```python
from build123d import *

# Parameters (mm, degrees)
SKETCH1_W                = 40
SKETCH1_H                = 40
BOSS_EXTRUDE1_DEPTH      = 40
SKETCH2_W                = 25
SKETCH2_H                = 20
CUT_EXTRUDE1_DEPTH       = 40
CHAMFER1_SIZE            = 15
CUT_EXTRUDE2_DEPTH       = 15
CHAMFER2_SIZE            = 4
SKETCH4_R                = 2.6
CUT_EXTRUDE3_DEPTH       = 17
BOSS_EXTRUDE2_DEPTH      = 8
BOSS_EXTRUDE2_DEPTH_BACK = 40
SKETCH5_W                = 40
SKETCH5_H                = 8.5
SKETCH10_W               = 14
SKETCH10_H               = 10
CUT_EXTRUDE5_DEPTH       = 26
SKETCH8_R                = 5.6
CUT_EXTRUDE4_DEPTH       = 34
BOSS_EXTRUDE3_DEPTH      = 20
FILLET3_R                = 4
FILLET4_R                = 2
CHAMFER7_SIZE            = 25
CHAMFER8_SIZE            = 2
CHAMFER8_SIZE2           = 10
FILLET7_R                = 2
SKETCH14_W               = 40
SKETCH14_H               = 8.5
BOSS_EXTRUDE4_DEPTH      = 15
SKETCH16_W               = 40
SKETCH16_H               = 8.5
BOSS_EXTRUDE5_DEPTH      = 15
SKETCH12_R               = 11.1
CUT_EXTRUDE6_DEPTH       = 4.5
CUT_EXTRUDE7_START       = -7.5
SKETCH13_R               = 11.1
CUT_EXTRUDE7_DEPTH       = 7.5
SKETCH15_R               = 2.1
CUT_EXTRUDE8_DEPTH       = 10
CHAMFER10_SIZE           = 0.5
FILLET8_R                = 8


with BuildPart() as part:
    # Sketch1 → Boss-Extrude1 (new body)
    with BuildSketch(Plane(origin=(0, 0, 0), x_dir=(1, 0, 0), z_dir=(0, 1, 0))):
        with Locations((20, 20)):
            Rectangle(SKETCH1_W, SKETCH1_H)
    extrude(amount=BOSS_EXTRUDE1_DEPTH)

    # Sketch2 → Cut-Extrude1 (cut)
    with BuildSketch(Plane(origin=(0, 40, 0), x_dir=(1, 0, 0), z_dir=(0, 1, 0))):
        with Locations((12.5, 30)):
            Rectangle(SKETCH2_W, SKETCH2_H)
    extrude(amount=-CUT_EXTRUDE1_DEPTH, mode=Mode.SUBTRACT)

    # Chamfer1
    chamfer1_edges = [part.edges().sort_by_distance(p)[0] for p in [
        (0, 20, 0),
    ]]
    chamfer(chamfer1_edges, length=CHAMFER1_SIZE)

    # Sketch3 → Cut-Extrude2 (cut)
    with BuildSketch(Plane.XY):
        Polygon((0, 10), (0, 15), (15, 15), (15, 5), (0, 5), align=None)
        Polygon((0, 30), (0, 25), (15, 25), (15, 35), (0, 35), align=None)
    extrude(amount=-CUT_EXTRUDE2_DEPTH, mode=Mode.SUBTRACT)

    # Chamfer2
    chamfer2_edges = [part.edges().sort_by_distance(p)[0] for p in [
        (15, 35, -7.5),
        (15, 25, -7.5),
        (15, 15, -7.5),
        (15, 5, -7.5),
    ]]
    chamfer(chamfer2_edges, length=CHAMFER2_SIZE)

    # Sketch4 → Cut-Extrude3 (cut)
    with BuildSketch(Plane.XY.offset(-15)):
        with Locations((8, 30)):
            Circle(SKETCH4_R)
        with Locations((8, 10)):
            Circle(SKETCH4_R)
    extrude(amount=-CUT_EXTRUDE3_DEPTH, mode=Mode.SUBTRACT)

    # Sketch5 → Boss-Extrude2 (add, two sides: drawn at the far end of the back side and taken through both)
    with BuildSketch(Plane(origin=(0, 0, -40), x_dir=(-1, 0, 0), z_dir=(0, 0, -1)).offset(-BOSS_EXTRUDE2_DEPTH_BACK)):
        with Locations((-60, 4.25)):
            Rectangle(SKETCH5_W, SKETCH5_H)
        with Locations((-60, 30.25)):
            Rectangle(SKETCH5_W, SKETCH5_H)
    extrude(amount=BOSS_EXTRUDE2_DEPTH + BOSS_EXTRUDE2_DEPTH_BACK)

    # Sketch10 → Cut-Extrude5 (cut)
    with BuildSketch(Plane(origin=(40, 0, 0), x_dir=(0, 0, -1), z_dir=(1, 0, 0))):
        with Locations((29, 20)):
            Rectangle(SKETCH10_W, SKETCH10_H)
    extrude(amount=-CUT_EXTRUDE5_DEPTH, mode=Mode.SUBTRACT)

    # Sketch8 → Cut-Extrude4 (cut)
    with BuildSketch(Plane(origin=(0, 32, 0), x_dir=(1, 0, 0), z_dir=(0, 1, 0))):
        with Locations(Location((65, 38, 0), (0, 0, 270))):
            Circle(SKETCH8_R)
    extrude(amount=-CUT_EXTRUDE4_DEPTH, mode=Mode.SUBTRACT)

    # Sketch9 → Boss-Extrude3 (add)
    with BuildSketch(Plane(origin=(40, 0, 0), x_dir=(0, 0, -1), z_dir=(1, 0, 0))):
        Polygon((0, 40), (0, 55), (4, 55), (20, 40), align=None)
        Polygon((0, 0), (0, -15), (4, -15), (20, 0), align=None)
    extrude(amount=-BOSS_EXTRUDE3_DEPTH)

    # Fillet3
    fillet3_edges = [part.edges().sort_by_distance(p)[0] for p in [
        (20, 55, -2),
        (40, 55, -2),
        (20, -15, -2),
        (40, -15, -2),
    ]]
    fillet(fillet3_edges, radius=FILLET3_R)

    # Fillet4
    fillet4_edges = [part.edges().sort_by_distance(p)[0] for p in [
        (32.5, 40, -40),
        (32.5, 0, -40),
    ]]
    fillet(fillet4_edges, radius=FILLET4_R)

    # Chamfer7
    chamfer7_edges = [part.edges().sort_by_distance(p)[0] for p in [
        (80, 4.25, 0),
        (80, 30.25, 0),
    ]]
    chamfer(chamfer7_edges, length=CHAMFER7_SIZE)

    # Chamfer8
    chamfer8_edges = [part.edges().sort_by_distance(p)[0] for p in [
        (40, 20, -36),
    ]]
    chamfer8_side = [part.faces().sort_by_distance(p)[0] for p in [
        (40, 16.5625, -17.75),
    ]]
    chamfer(chamfer8_edges, length=CHAMFER8_SIZE, length2=CHAMFER8_SIZE2, reference=chamfer8_side[0])

    # Fillet7
    fillet7_edges = [part.edges().sort_by_distance(p)[0] for p in [
        (27.5, 15, -36),
        (32.5, 15, -22),
        (32.5, 25, -22),
        (27.5, 25, -36),
        (35, 25, -37),
        (35, 15, -37),
    ]]
    fillet(fillet7_edges, radius=FILLET7_R)

    # Sketch14 → Boss-Extrude4 (add)
    with BuildSketch(Plane(origin=(0, 0, -48), x_dir=(-1, 0, 0), z_dir=(0, 0, -1))):
        with Locations((-60, 4.25)):
            Rectangle(SKETCH14_W, SKETCH14_H)
    extrude(amount=BOSS_EXTRUDE4_DEPTH)

    # Sketch16 → Boss-Extrude5 (add)
    with BuildSketch(Plane(origin=(0, 0, -48), x_dir=(-1, 0, 0), z_dir=(0, 0, -1))):
        with Locations((-60, 30.25)):
            Rectangle(SKETCH16_W, SKETCH16_H)
    extrude(amount=BOSS_EXTRUDE5_DEPTH)

    # Sketch12 → Cut-Extrude6 (cut)
    with BuildSketch(Plane(origin=(0, 34.5, 0), x_dir=(1, 0, 0), z_dir=(0, 1, 0))):
        with Locations(Location((65, 38, 0), (0, 0, 180))):
            Circle(SKETCH12_R)
    extrude(amount=-CUT_EXTRUDE6_DEPTH, mode=Mode.SUBTRACT)

    # Sketch13 → Cut-Extrude7 (cut)
    with BuildSketch(Plane.XZ.offset(CUT_EXTRUDE7_START)):
        with Locations(Location((65, -38, 0), (0, 0, 180))):
            Circle(SKETCH13_R)
    extrude(amount=CUT_EXTRUDE7_DEPTH, mode=Mode.SUBTRACT)

    # Sketch15 → Cut-Extrude8 (cut)
    with BuildSketch(Plane.XZ):
        with Locations(Location((65.260929409, -54.130501699, 0), (0, 0, 270))):
            Circle(SKETCH15_R)
        with Locations(Location((65.16900186, -21.868239994, 0), (0, 0, 270))):
            Circle(SKETCH15_R)
    extrude(amount=-CUT_EXTRUDE8_DEPTH, mode=Mode.SUBTRACT)

    # Chamfer10
    chamfer10_edges = [part.edges().sort_by_distance(p)[0] for p in [
        (76.1, 34.5, -38),
        (76.1, 0, -38),
    ]]
    chamfer(chamfer10_edges, length=CHAMFER10_SIZE)

    # Fillet8
    fillet8_edges = [part.edges().sort_by_distance(p)[0] for p in [
        (55, 30.25, 0),
        (55, 4.25, 0),
        (80, 4.25, -25),
        (80, 30.25, -25),
        (80, 4.25, -63),
        (40, 4.25, -63),
        (80, 30.25, -63),
        (40, 30.25, -63),
    ]]
    fillet(fillet8_edges, radius=FILLET8_R)


solid = part.part
```
Geometry: final body of the model. Coordinates: model frame, mm. A direction names the side the tool comes from. Round coordinates to 2 decimals unless told otherwise and drop trailing zeros. Loops run counter-clockwise (first coordinate to the right, second up) from the corner with the lowest first, then second, coordinate; pieces in that order, holes last. Notation, with made-up numbers: (67, 89) -> (80, 89) arc R14 ccw to (80, 106) -> close; hole circle Ø5 at (34.25, 51). An arc over 180 degrees is marked (long way). Write each question's results on one line, items separated by ' | '.
Item 1: Pin query (flat end, axial travel): pin 1 Ø2.5 at (x, z) = (65.26, -54.13) entering from -Y; pin 2 Ø5.5 at (x, z) = (5.5, -7.5) entering from +Y; pin 3 Ø6 at (x, y) = (70, -4.5) entering from -Z; pin 4 Ø20 at (x, z) = (64.5, -45.5) entering from -Y. Return the tip coordinate at first contact, or that it passes through.
Answers below:
pin 1: stops at y = 26 | pin 2: stops at y = 40 | pin 3: passes through | pin 4: stops at y = 0
Item 2: Cut plane C-C on x = 69.5. State how many separate pieces and enclosed holes the cut face has, and give its area (3 significant figures).
Answers below:
separate pieces: 4 | enclosed holes: 0 | area: 547 mm²
Item 3: Cut plane D-D on y = 42.5. Return the cut outline in (x, z), and give its area (3 significant figures).
Answers below:
outline: (20, -17.33) -> (40, -17.33) -> (40, 0) -> (20, 0) -> close | area: 347 mm²
Item 4: Cut plane A-A on y = 10. Return the cut outline in (x, z).
Answers below:
outline: (0, -20) -> (5.4, -20) -> (5.4, -15) -> (0, -15) -> close; (10.6, -20) -> (25, -20) -> (25, -40) -> (40, -40) -> (40, 0) -> (15, 0) -> (15, -15) -> (10.6, -15) -> close
Item 5: Pull-direction query (Z, two-part tool) for faces 5 (the face through (67.25, 4.19, -21.59)), 6 (the face through (13, 27, -9)), 7 (the face through (8, 20, -7)), 8 (the face through (68, 30, -33)); classes: pulls with the +Z half, pulls with the -Z half, needs draft (parallel to the pull), parting line crosses it, or undercut.
Answers below:
face 5: undercut | face 6: needs draft | face 7: pulls with the +Z half | face 8: undercut
Item 6: Line query: probe 1 along Y at (x, z) = (8, -17); probe 2 along Y at (x, z) = (63.5, -58); probe 3 along Y at (x, z) = (67, -47). Output: solid intervals per line, ascending. Write a range as [from, to].
Answers below:
probe 1: y = [0, 7.4], [12.6, 27.4], [32.6, 40] | probe 2: y = [0, 8.5], [26, 34.5] | probe 3: y = [7.5, 8.5], [26, 30]
Item 7: Set-up query: faces 1 (the face through (8, 15, -12)), 2 (the face through (79.408, 30.31, -25.293)), 3 (the face through (40, 15, -15)), 4 (the face through (32.61, 0.57, -39.4)). Return all of +Z, -Z, +X, -X, +Y, -Y with unobstructed straight access to the full face (end or side cutting, diameter ignored); none if empty.
Answers below:
face 1: +Z, -X | face 2: +Z, +X, +Y, -Y | face 3: +Z, -Z, +X | face 4: -Z, -X, -Y
Item 8: Cut plane B-B on x = 8. Return the cut outline in (y, z), and give its area (3 significant figures).
Answers below:
outline: (0, -20) -> (7.4, -20) -> (7.4, -15) -> (5, -15) -> (5, -7) -> (0, -7) -> close; (12.6, -20) -> (27.4, -20) -> (27.4, -15) -> (25, -15) -> (25, -7) -> (15, -7) -> (15, -15) -> (12.6, -15) -> close; (32.6, -20) -> (40, -20) -> (40, -7) -> (35, -7) -> (35, -15) -> (32.6, -15) -> close | area: 308 mm²
